from build123d import *

# Parameters (mm, degrees)
F1_DEPTH    = 20
F2_R        = 19.5
F2_R_2      = 16.2
F3_DEPTH    = 3
F4_T1_DEPTH = 51.8336597593
F4_T3_DEPTH = 51.8336597593


# Not quite as in the source:
# - a fillet or chamfer that OpenCascade refuses, or shapes differently, is made with other operations: its cross-section is extruded or revolved along the edge and cut away or added


with BuildPart() as f1:
    # F0 (on Top) → F1 (new body)
    with BuildSketch(Plane.XY):
        with BuildLine():
            ThreePointArc((15.7618937877, -3.7420187366), (8.4993351577, -13.7913488056), (-3.7420187366, -15.7618937877))
            Line((-3.7420187366, -15.7618937877), (-3.8344142609, -16.1510763504))
            ThreePointArc((-3.8344142609, -16.1510763504), (8.709195285, -14.1318759366), (16.1510763504, -3.8344142609))
            Line((16.1510763504, -3.8344142609), (15.7618937877, -3.7420187366))
        make_face()
    extrude(amount=F1_DEPTH)

    # F2 (on Top) → F3 (join)
    with BuildSketch(Plane.XY):
        Circle(F2_R)
        Circle(F2_R_2, mode=Mode.SUBTRACT)
    extrude(amount=-F3_DEPTH)

    # F4: chamfer of 10 on 2 edges, made by hand

    # F4_s2 → F4_t1 (cut)
    with BuildSketch(Plane(origin=(41.1724307405, -9.7747142149, 0), x_dir=(0, 0, 1), z_dir=(-0.9729564066, 0.2309888109, 0))):
        Polygon((10, 0), (20, -10), (20, 0), align=None)
    extrude(amount=F4_T1_DEPTH, mode=Mode.SUBTRACT)

    # F4_s4 → F4_t3 (cut)
    with BuildSketch(Plane(origin=(2.1982812174, 9.2594606024, 0), x_dir=(0, 0, 1), z_dir=(-0.2309888109, -0.9729564066, 0))):
        Polygon((10, 0), (20, -10), (20, 0), align=None)
    extrude(amount=F4_T3_DEPTH, mode=Mode.SUBTRACT)


solid = f1.part
Geometry: final body of the model. Coordinates: model frame, mm. A direction names the side the tool comes from. Coordinates: 2 decimals unless noted, no trailing zeros. Loops run counter-clockwise (first coordinate to the right, second up) from the corner with the lowest first, then second, coordinate; pieces in that order, holes last. Notation, with made-up numbers: (5.5, 46.25) - (59.5, 46.25) arc R18 ccw to (59.5, 77.25) - close; hole circle Ø11 at (-13, 18). An arc over 180 degrees is marked (long way). One line per question, with ' | ' between items. Start each with the question number.
(1) Cut plane D-D on z = 7.75. Output: boundary loops of the cut face in (x, y).
(2) Cut plane A-A on y = 0. Output: boundary loops of the cut face in (x, z).
(3) Cut plane B-B on x = 7.5. Output: boundary loops of the cut face in (y, z).
(4) First-contact query: pin 1 (1.5 mm diameter, centred on x = 15.5, y = -2, fed in from +Z); pin 2 (2 mm diameter, centred on x = -1, z = 10.5, fed in from -Y); pin 3 (1 mm diameter, centred on y = -12.5, z = 7.5, fed in from +X). Flat tips, straight axial feed; report the tip coordinate or a pass-through.
(5) Ray query, L1, parallel to Y at x = 0, z = -1.5; L2, parallel to Z at x = 7, y = 15; L3, parallel to X at y = 2.5, z = -2. Return the intervals inside material, ascending. Write a range as from..to.
(6) Reachability of faces 1 (the flat face through (8.62, -13.93, 20)), 2 (the flat face through (-7, 15, 0)) from +Z, -Z, +X, -X, +Y, -Y: full face, straight path, thin tool, end or side. Return the list, or none.
(7) Cut plane C-C on x = 0. Output: boundary loops of the cut face in (y, z).
Here are the results:
1) outline: (-3.83, -16.15) arc R16.6 ccw to (16.15, -3.83) - (15.76, -3.74) arc R16.2 cw to (-3.74, -15.76) - close
2) outline: (-19.5, -3) - (-16.2, -3) - (-16.2, 0) - (-19.5, 0) - close; (16.2, -3) - (19.5, -3) - (19.5, 0) - (16.2, 0) - close
3) outline: (-18, -3) - (-14.36, -3) - (-14.36, 20) - (-14.81, 20) - (-14.81, 0) - (-18, 0) - close; (14.36, -3) - (18, -3) - (18, 0) - (14.36, 0) - close
4) pin 1: z = 0 | pin 2: y = -16.6 | pin 3: x = 11.47
5) L1: -19.5..-16.2, 16.2..19.5 | L2: -3..0 | L3: -19.34..-16.01, 16.01..19.34
6) face 1: +Z, +X, -X, +Y, -Y | face 2: +Z
7) outline: (-19.5, -3) - (-16.2, -3) - (-16.2, 13.74) - (-16.6, 13.83) - (-16.6, 0) - (-19.5, 0) - close; (16.2, -3) - (19.5, -3) - (19.5, 0) - (16.2, 0) - close
